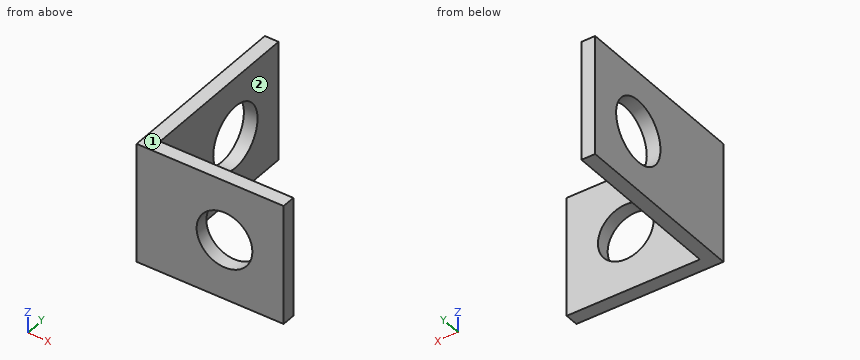
Autodesk Inventor part; units mm, degrees
ref_plane "YZ Plane" through (0, 0, 0) normal (1, 0, 0) x (0, 1, 0)
ref_plane "XZ Plane" through (0, 0, 0) normal (0, 1, 0) x (-1, 0, 0)
ref_plane "XY Plane" through (0, 0, 0) normal (0, 0, 1) x (1, 0, 0)
sketch "Sketch1" plane through (0, 0, 0) normal (0, 0, 1) x (1, 0, 0)
  line L0 (0, 0) -> (7.89, 0)
  line L1 (7.89, 0) -> (7.89, -0.81)
  line L2 (7.89, -0.81) -> (-0.81, -0.81)
  line L3 (-0.81, -0.81) -> (-0.81, 9.89)
  line L4 (-0.81, 9.89) -> (0, 9.89)
  line L5 (0, 9.89) -> (0, 0)
  dimension "d0" = 7.89
  dimension "d1" = 0.81
  dimension "d2" = 8.7
  dimension "d3" = 10.7
extrude "Extrusion1" add sketch "Sketch1" against normal blind 7.1
sketch "Sketch2" plane through (0, 0, 0) normal (0, 1, 0) x (1, 0, 0)
  line L0 (0, 0) -> (-0.81, 0)
  line L1 (-0.81, 7.1) -> (0, 7.1)
  line L2 (-0.81, 0) -> (-0.81, 7.1)
  line L3 (-0.81, 0) -> (-0.81, 7.1)
  line L4 (-0.81, 3.55) -> (4.39, 3.55)
  circle A0 centre (4.39, 3.55) radius 1.65
  dimension "d6" = 5.2
  dimension "d7" = 3.3
extrude "Extrusion2" cut sketch "Sketch2" against normal blind 7.1
sketch "Sketch3" plane through (0, 0, 0) normal (1, 0, 0) x (0, 0, -1)
  line L0 (0, -0.81) -> (7.1, -0.81)
  line L1 (3.55, -0.81) -> (3.55, 6.29)
  circle A0 centre (3.55, 6.29) radius 1.85
  point P0 (0, 0)
  dimension "d10" = 7.1
  dimension "d11" = 3.7
extrude "Extrusion3" cut sketch "Sketch3" against normal blind 7.1
properties part number "615Bracket"
Geometry check sheet. Reference: the model listing, model coordinates, mm. Face numbers are marked on the shaded views. A direction names the side the tool comes from. Round coordinates to 2 decimals unless told otherwise and drop trailing zeros. Write each loop counter-clockwise with the first axis right and the second up, starting at its lowest first coordinate (ties: lowest second). Pieces come first, ordered by that corner, then holes. Notation, with made-up numbers: (-32.75, -18.75) - (26.25, -18.75) arc R28 cw to (26.25, 20.25) - close; hole circle Ø9 at (14.25, 82.5). An arc over 180 degrees is marked (long way). One line per item, written item: value.
1. Cross-section at D-D on z = -2.75. Record the boundary of the cut face in (x, y), and give its area (3 significant figures).
The answers:
outline: (-0.81, -0.81) - (2.95, -0.81) - (2.95, 0) - (0, 0) - (0, 4.62) - (-0.81, 4.62) - close; (-0.81, 7.96) - (0, 7.96) - (0, 9.89) - (-0.81, 9.89) - close; (5.83, -0.81) - (7.89, -0.81) - (7.89, 0) - (5.83, 0) - close
area: 10.0 mm^2
2. Cross-section at B-B on z = -3.55. Record the boundary of the cut face in (x, y).
The answers:
outline: (-0.81, -0.81) - (2.74, -0.81) - (2.74, 0) - (0, 0) - (0, 4.44) - (-0.81, 4.44) - close; (-0.81, 8.14) - (0, 8.14) - (0, 9.89) - (-0.81, 9.89) - close; (6.04, -0.81) - (7.89, -0.81) - (7.89, 0) - (6.04, 0) - close
3. Set-up check for the marked faces 1 and 2: record each of +Z, -Z, +X, -X, +Y, -Y from which the full face is reachable in a straight line by a thin tool's end or side.
The answers:
face 1: +Z, +X, -X, +Y, -Y
face 2: +Z, -Z, +X, +Y
4. Depth check by flat-ended pin: pin 1 Ø2 at (y, z) = (3.5, -4.5) entering from +X. Enter the tip coordinate at first touch or a pass-through.
The answers:
pin 1: stops at x = 0
5. Scan lines: L1, parallel to Y at x = -0.5, z = -3.55; L2, parallel to Z at x = 4.39, y = -0.35; L3, parallel to Y at x = 4, z = -1. Record each from-to range of solid material in increasing order.
The answers:
L1: y = -0.81 to 4.44, 8.14 to 9.89
L2: z = -7.1 to -5.2, -1.9 to 0
L3: y = -0.81 to 0
6. Cross-section at A-A on y = 5.25. Record the boundary of the cut face in (x, z), and give its area (3 significant figures).
The answers:
outline: (-0.81, -7.1) - (0, -7.1) - (0, -5.08) - (-0.81, -5.08) - close; (-0.81, -2.02) - (0, -2.02) - (0, 0) - (-0.81, 0) - close
area: 3.27 mm^2
7. Cross-section at C-C on x = 4.5. Record the boundary of the cut face in (y, z).
The answers:
outline: (-0.81, -7.1) - (0, -7.1) - (0, -5.2) - (-0.81, -5.2) - close; (-0.81, -1.9) - (0, -1.9) - (0, 0) - (-0.81, 0) - close
